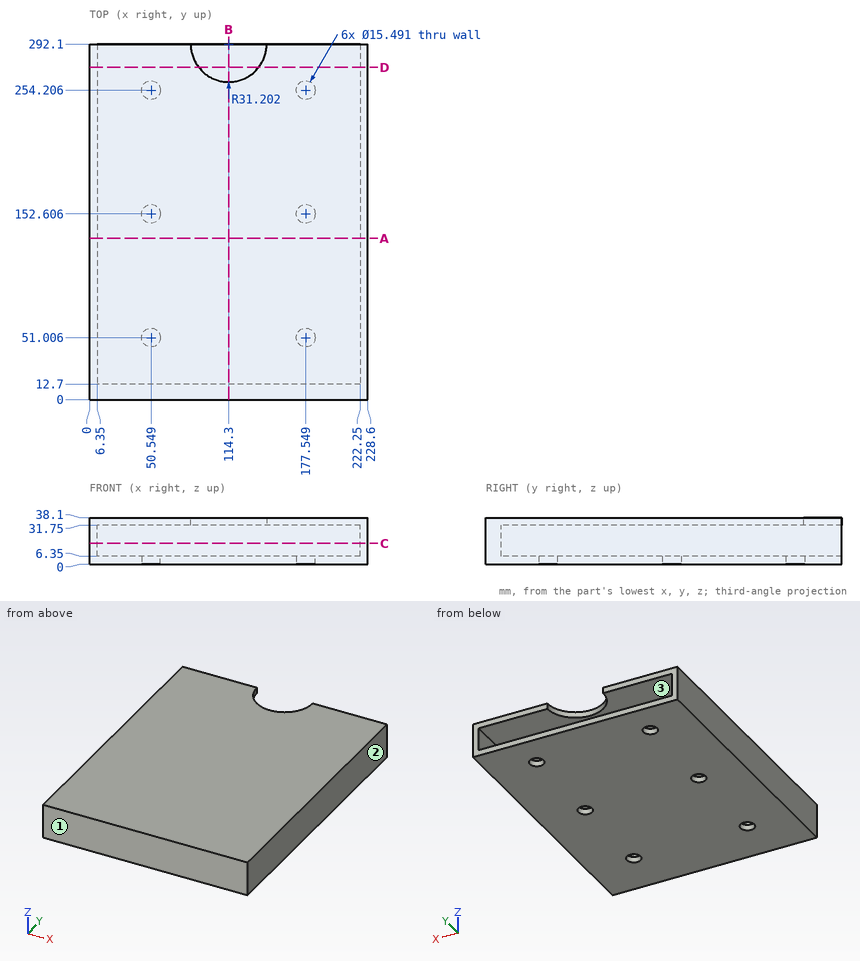
Print and shaded views of the part. All mm, measured from the part's lowest x, y and z. Give positions to 0.01 mm unless a question says otherwise; leave off trailing zeros. Write each loop counter-clockwise with the first axis right and the second up, starting at its lowest first coordinate (ties: lowest second). Pieces come first, ordered by that corner, then holes. Notation, with made-up numbers: M -7.75,-33 L 23.25,-33 A14 cw 23.25,-12 Z; hole C -22.5,79 d11. An arc over 180 degrees is marked long. Use a Markdown table: item, result.
1) Cut at C-C (z = 17). List the corners of the cut face in (x, y).
Responses:
| item | result |
|---|---|
| outline | M 0,0 L 228.6,0 L 228.6,292.1 L 222.25,292.1 L 222.25,12.7 L 6.35,12.7 L 6.35,292.1 L 0,292.1 Z |
2) Pull direction X, two halves, no side cores. Call the marked faces 1, 2 and 3: +X half, -X half, draft (parallel to the pull), parting line (faces both ways), or undercut.
Responses:
| item | result |
|---|---|
| face 1 | draft |
| face 2 | +X half |
| face 3 | undercut |
3) Cut at A-A (y = 132.5). List the corners of the cut face in (x, z).
Responses:
| item | result |
|---|---|
| outline | M 0,0 L 228.6,0 L 228.6,38.1 L 0,38.1 Z; hole M 6.35,6.35 L 222.25,6.35 L 222.25,31.75 L 6.35,31.75 Z |
4) Cut at B-B (x = 114.3). List the corners of the cut face in (y, z).
Responses:
| item | result |
|---|---|
| outline | M 0,0 L 292.1,0 L 292.1,6.35 L 12.7,6.35 L 12.7,31.75 L 260.9,31.75 L 260.9,38.1 L 0,38.1 Z |
5) Pin check, flat tips, straight feed: pin 1 (14 mm diameter, centred on x = 177.55, y = 254.21, fed in from -Z); pin 2 (2 mm diameter, centred on x = 134, z = 16.5, fed in from +Y). Stop position of each tip, or through.
Responses:
| item | result |
|---|---|
| pin 1 | stops at z = 31.75 |
| pin 2 | stops at y = 12.7 |
6) Cut at D-D (y = 273). List the corners of the cut face in (x, z), and give its area (3 significant figures).
Responses:
| item | result |
|---|---|
| outline | M 0,0 L 228.6,0 L 228.6,38.1 L 138.97,38.1 L 138.97,31.75 L 222.25,31.75 L 222.25,6.35 L 6.35,6.35 L 6.35,31.75 L 89.63,31.75 L 89.63,38.1 L 0,38.1 Z |
| area | 2,910 mm2 |
7) Drill centre lines: line 1 (X direction, y = 222, z = 7.5); line 2 (Z direction, x = 17.5, y = 62); line 3 (Y direction, x = 165.5, z = 31.5). Where is each one in solid material? Low to high. Write a range as from..to.
Responses:
| item | result |
|---|---|
| line 1 | x = 0..6.35, 222.25..228.6 |
| line 2 | z = 0..6.35, 31.75..38.1 |
| line 3 | y = 0..12.7 |
